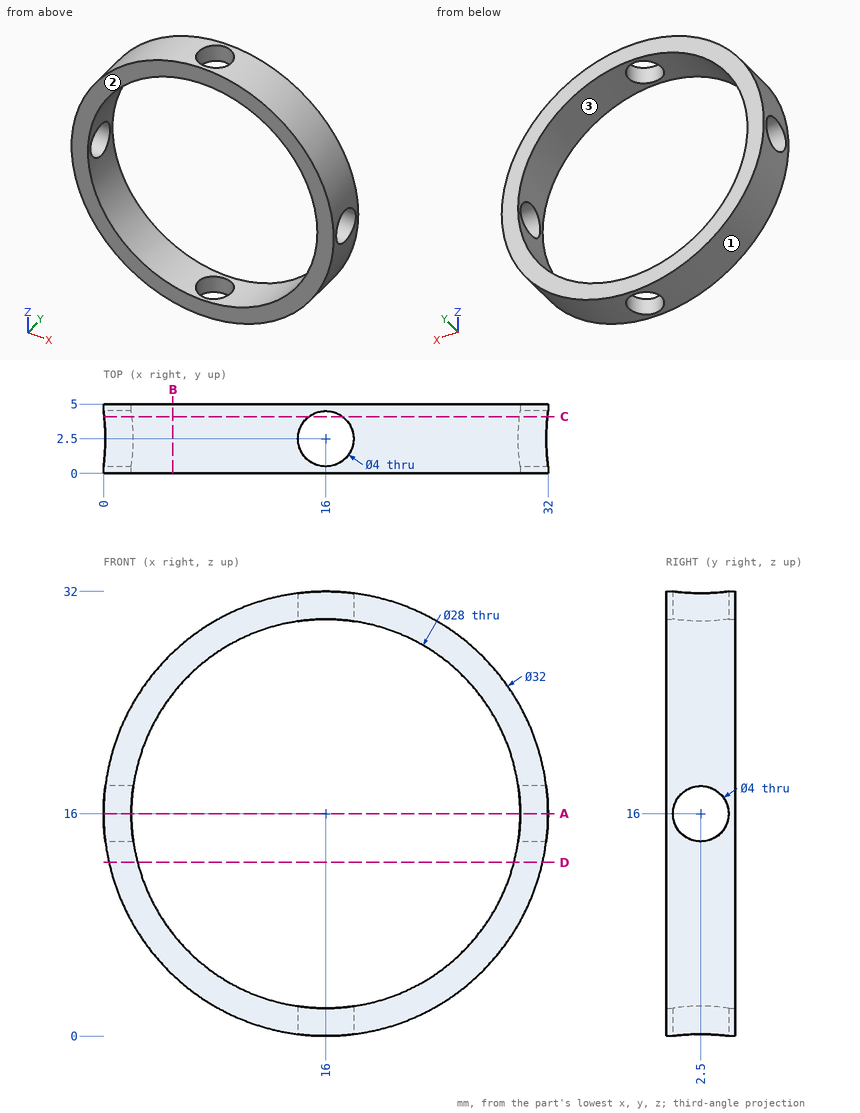
Drawing for the job (mm, zero at the part's lowest x, y, z). Give positions to 0.01 mm unless a question says otherwise; leave off trailing zeros. Order: outer loops, then holes, each group sorted by start corner. A loop starts at its lowest first (then second) coordinate and runs counter-clockwise, first axis right, second up. Notation, with made-up numbers: M 2,31.5 L 15,31.5 A24 cw 15,63.5 Z; hole C 73,13 d7. An arc over 180 degrees is marked long. Use a Markdown table: item, result. Add a question column.
(1) Saw through at C-C, the plane y = 4.1. Give the cut face in (x, z).
(2) Mould opens along Z. For the marked faces 1, 2 and 3 say: +Z half, -Z half, draft (parallel to the pull), parting line (faces both ways), or undercut.
(3) Saw through at A-A, the plane z = 16. Give the cut face in (x, y).
(4) Saw through at B-B, the plane x = 5. Give the cut face in (y, z).
(5) Drop flat-ended pins along their axis: P1, Ø1.5, axis at x = 18.5, y = 4.5, coming from the +Z side; P2, Ø1, axis at x = 6.5, z = 23, coming from the +Y side (3 decimals). Give the stop position or say it passes through.
(6) Probe line 1 along X through (y, z) = (3.5, 12); line 2 along X through (y, z) = (4.6, 5); line 3 along Y through (x, z) = (16, 30.5). List the from-to ranges inside material, lowest first. Write a range as [from, to].
(7) Saw through at D-D, the plane z = 12.5. Give the cut face in (x, y).
Answer key:
| question | item | result |
|---|---|---|
| 1 | outline | M 0.05,14.8 A16 ccw 14.8,0.05 L 14.8,2.05 A14 cw 2.05,14.8 Z; M 0.05,17.2 L 2.05,17.2 A14 cw 14.8,29.95 L 14.8,31.95 A16 ccw Z; M 17.2,0.05 A16 ccw 31.95,14.8 L 29.95,14.8 A14 cw 17.2,2.05 Z; M 17.2,29.95 A14 cw 29.95,17.2 L 31.95,17.2 A16 ccw 17.2,31.95 Z |
| 2 | face 1 | parting line |
| 2 | face 2 | draft |
| 2 | face 3 | undercut |
| 3 | outline | M 0,0 L 2,0 L 2,0.5 L 0,0.5 Z; M 0,4.5 L 2,4.5 L 2,5 L 0,5 Z; M 30,0 L 32,0 L 32,0.5 L 30,0.5 Z; M 30,4.5 L 32,4.5 L 32,5 L 30,5 Z |
| 4 | outline | M 0,4.38 L 5,4.38 L 5,7.34 L 0,7.34 Z; M 0,24.66 L 5,24.66 L 5,27.62 L 0,27.62 Z |
| 5 | P1 | z = 31.9 |
| 5 | P2 | through |
| 6 | line 1 | [0.51, 2.58], [29.42, 31.49] |
| 6 | line 2 | [4.38, 7.34], [24.66, 27.62] |
| 6 | line 3 | [0, 0.5], [4.5, 5] |
| 7 | outline | M 0.39,0 L 2.44,0 L 2.44,5 L 0.39,5 Z; M 29.56,0 L 31.61,0 L 31.61,5 L 29.56,5 Z |
